```python
from build123d import *

# Parameters (mm, degrees)
F0_W     = 48
F0_H     = 25
F1_DEPTH = 10
F3_DEPTH = 15
F4_DEPTH = 20
F5_W     = 20
F5_H     = 10
F6_DEPTH = 48


with BuildPart() as f1:
    # F0 (on Front) → F1 (new body)
    with BuildSketch(Plane.XZ):
        Rectangle(F0_W, F0_H)
    extrude(amount=-F1_DEPTH)

    # F2 (on face) → F3 (cut)
    with BuildSketch(Plane.XY.offset(12.5)):
        Polygon((-24, 0), (-10, 0), (-4, 10), (-24, 10), align=None)
        Polygon((4, 10), (10, 0), (24, 0), (24, 10), align=None)
    extrude(amount=-F3_DEPTH, mode=Mode.SUBTRACT)

    # F0 (on Front) → F4 (join)
    with BuildSketch(Plane.XZ):
        Rectangle(F0_W, F0_H)
    extrude(amount=F4_DEPTH)

    # F5 (on face) → F6 (cut)
    with BuildSketch(Plane.YZ.offset(24)):
        with Locations((0, -7.5)):
            Rectangle(F5_W, F5_H)
    extrude(amount=-F6_DEPTH, mode=Mode.SUBTRACT)


solid = f1.part
```
The model under review builds one solid part; all positions refer to its coordinate system, in mm. A direction names the side the tool comes from. Coordinates: 2 decimals unless noted, no trailing zeros. Write each loop counter-clockwise with the first axis right and the second up, starting at its lowest first coordinate (ties: lowest second). Pieces come first, ordered by that corner, then holes. Notation, with made-up numbers: (86.5, 74.5) -> (144.5, 74.5) arc R25 cw to (144.5, 113.5) -> close; hole circle Ø9 at (-39, -2). An arc over 180 degrees is marked (long way). One line per item, written item: value. Start each with the question number.
Q1. To check wall thickness, follow probe 1 along Z at (x, y) = (3.5, -9.5); probe 2 along Y at (x, z) = (-12.5, 8.75); probe 3 along Y at (x, z) = (-11, -7.75). State the ranges of each line that lie inside material, in increasing order.
Q2. Add section A-A, the plane z = 7. Give the boundary of the cut face in (x, y), then the cut area to 3 significant figures.
Q3. For faces 1 (the face through (-17, 0, 5)), 2 (the face through (17, 0, 5)), 3 (the face through (0, -2, -2.5)), list the 3-axis set-ups (+Z, -Z, +X, -X, +Y, -Y) from which the entire face can be reached by the end or side of a thin tool; tool diameter is ignored.
Q4. Add section C-C, the plane y = 5.75. Give the boundary of the cut face in (x, z), then the cut area to 4 significant figures.
Q5. Add section B-B, the plane x = -10.5. Give the boundary of the cut face in (y, z).
Q6. Add section D-D, the plane z = -4. Give the boundary of the cut face in (x, y).
Q7. Clearance check with flat-ended pins moving along their axes: P1, Ø6, axis at x = 2.5, y = 0, coming from the -Z side; P2, Ø11, axis at x = 9, z = -9, coming from the +Y side; P3, Ø7, axis at x = -16, z = 8, coming from the +Y side. State where each tip first meets the part, or that it passes through.
Response:
1. probe 1: -2.5 to 12.5
1. probe 2: -20 to 0
1. probe 3: -20 to -10
2. outline: (-24, -20) -> (24, -20) -> (24, 0) -> (10, 0) -> (4, 10) -> (-4, 10) -> (-10, 0) -> (-24, 0) -> close
2. area: 1,100 mm²
3. face 1: +Z, -Z, -X, +Y
3. face 2: +Z, -Z, +X, +Y
3. face 3: -Z, +X, -X, +Y
4. outline: (-6.55, -2.5) -> (6.55, -2.5) -> (6.55, 12.5) -> (-6.55, 12.5) -> close
4. area: 196.5 mm²
5. outline: (-20, -12.5) -> (-10, -12.5) -> (-10, -2.5) -> (0, -2.5) -> (0, 12.5) -> (-20, 12.5) -> close
6. outline: (-24, -20) -> (24, -20) -> (24, -10) -> (-24, -10) -> close
7. P1: z = -2.5
7. P2: y = -10
7. P3: y = 0
